```python
from build123d import *

# Parameters (mm, degrees)
F0_R     = 1.2446
F1_DEPTH = 2.921
F0_W     = 3.8608
F0_H     = 4.4704
F2_DEPTH = 2.54
F3_DEPTH = 2.921
F4_DEPTH = 2.54
F5_R     = 1.2446
F6_DEPTH = 6.35


with BuildPart() as f1:
    # F0 (on Front) → F1 (new body)
    with BuildSketch(Plane.XZ):
        with BuildLine():
            Line((0, 4.4704), (0.8382, 4.4704))
            Line((0.8382, 4.4704), (4.699, 4.4704))
            Line((4.699, 4.4704), (5.5372, 4.4704))
            Line((5.5372, 4.4704), (5.5372, 6.5786))
            ThreePointArc((5.5372, 6.5786), (2.7686, 9.3472), (0, 6.5786))
            Line((0, 6.5786), (0, 4.4704))
        make_face()
        with Locations((2.7686, 6.3246)):
            Circle(F0_R, mode=Mode.SUBTRACT)
    extrude(amount=F1_DEPTH)

    # F0 (on Front) → F2 (join)
    with BuildSketch(Plane.XZ):
        with Locations((2.7686, 2.2352)):
            Rectangle(F0_W, F0_H)
    extrude(amount=F2_DEPTH)

    # F0 (on Front) → F3 (join)
    with BuildSketch(Plane.XZ):
        with BuildLine():
            Line((0, 4.4704), (0.8382, 4.4704))
            Line((0.8382, 4.4704), (4.699, 4.4704))
            Line((4.699, 4.4704), (5.5372, 4.4704))
            Line((5.5372, 4.4704), (5.5372, 6.5786))
            ThreePointArc((5.5372, 6.5786), (2.7686, 9.3472), (0, 6.5786))
            Line((0, 6.5786), (0, 4.4704))
        make_face()
        with Locations((2.7686, 6.3246)):
            Circle(F0_R, mode=Mode.SUBTRACT)
    extrude(amount=-F3_DEPTH)

    # F0 (on Front) → F4 (join)
    with BuildSketch(Plane.XZ):
        with Locations((2.7686, 2.2352)):
            Rectangle(F0_W, F0_H)
    extrude(amount=-F4_DEPTH)

    # F5 (on face) → F6 (cut)
    with BuildSketch(Plane(origin=(0, 0, 0), x_dir=(1, 0, 0), z_dir=(0, 0, -1))):
        with Locations((2.7686, 0)):
            Circle(F5_R)
    extrude(amount=-F6_DEPTH, mode=Mode.SUBTRACT)


solid = f1.part
```
Geometry check sheet. Reference: the model listing, model coordinates, mm. A direction names the side the tool comes from. Coordinates: 2 decimals unless noted, no trailing zeros. Order: outer loops, then holes, each group sorted by start corner. A loop starts at its lowest first (then second) coordinate and runs counter-clockwise, first axis right, second up. Notation, with made-up numbers: M -2.75,-29 L 28.25,-29 A20 ccw 28.25,-15 Z; hole C 3,72 d1. An arc over 180 degrees is marked long. One line per question, with ' | ' between items. Start each with the question number.
Item 1: Cross-section at D-D on z = 1. Enter the section's corners in (x, y), then the cut area to 3 significant figures.
Item 2: Cross-section at C-C on x = 3.7. Enter the section's corners in (y, z).
Item 3: Cross-section at B-B on y = -1.7. Enter the section's corners in (x, z), then the cut area to 3 significant figures.
Item 4: Set-up check for faces 1 (the flat face through (4.699, 0, 2)), 2 (the flat face through (0.838, 0, 2)), 3 (the flat face through (3, -2.54, 2)): record each of +Z, -Z, +X, -X, +Y, -Y from which the full face is reachable in a straight line by a thin tool's end or side.
Item 5: Draft check along Y on faces 4 (the cylindrical face through (2.607, -1.234, 2.415)), 5 (the flat face through (3, 2.54, 2)), 6 (the cylindrical face through (2.61, -0.04, 7.56)). Enter one of: pulls with the +Y half, pulls with the -Y half, needs draft (parallel to the pull), parting line crosses it, or undercut.
Item 6: Cross-section at A-A on z = 5.5. Enter the section's corners in (x, y), then the cut area to 3 significant figures.
Item 7: Material ranges on L1, parallel to X at y = 0, z = 3; L2, parallel to Z at x = 3.85, y = -2.05; L3, parallel to X at y = -2.5, z = 3.5, recorded low to high. Write a range as [from, to].
Item 8: Gauge pin test, flat ends, axial feed: pin 1 (3.5 mm diameter, centred on y = 0.5, z = 3, fed in from -X); pin 2 (1.2 mm diameter, centred on x = 2, z = 3.5, fed in from +Y); pin 3 (3 mm diameter, centred on y = 0.5, z = 2, fed in from -X). Record the tip position at first contact, or that the pin passes through.
Findings:
1) outline: M 0.84,-2.54 L 4.7,-2.54 L 4.7,2.54 L 0.84,2.54 Z; hole C 2.77,0 d2.49 | area: 14.7 mm²
2) outline: M -2.92,4.47 L -2.54,4.47 L -2.54,0 L -0.83,0 L -0.83,5.5 L -2.92,5.5 Z; M -2.92,7.15 L 2.92,7.15 L 2.92,9.19 L -2.92,9.19 Z; M 0.83,0 L 2.54,0 L 2.54,4.47 L 2.92,4.47 L 2.92,5.5 L 0.83,5.5 Z
3) outline: M 0,4.47 L 0.84,4.47 L 0.84,0 L 4.7,0 L 4.7,4.47 L 5.54,4.47 L 5.54,6.58 A2.77 ccw 0,6.58 Z; hole C 2.77,6.32 d2.49 | area: 36.1 mm²
4) face 1: -Z, +X, +Y, -Y | face 2: -Z, -X, +Y, -Y | face 3: -Z, +X, -X, -Y
5) face 4: undercut | face 5: pulls with the +Y half | face 6: needs draft
6) outline: M 0,-2.92 L 1.84,-2.92 L 1.84,-0.82 A1.24 cw 1.84,0.82 L 1.84,2.92 L 0,2.92 Z; M 3.7,-2.92 L 5.54,-2.92 L 5.54,2.92 L 3.7,2.92 L 3.7,0.82 A1.24 cw 3.7,-0.82 Z | area: 20.7 mm²
7) L1: x = [0.84, 1.52], [4.01, 4.7] | L2: z = [0, 5.71], [6.94, 9.13] | L3: x = [0.84, 4.7]
8) pin 1: stops at x = 0 | pin 2: stops at y = 2.54 | pin 3: stops at x = 0.84
